For this review, take the finished solid that the model builds, in its own axes (mm). A direction names the side the tool comes from. Round coordinates to 2 decimals unless told otherwise and drop trailing zeros. Write each loop counter-clockwise with the first axis right and the second up, starting at its lowest first coordinate (ties: lowest second). Pieces come first, ordered by that corner, then holes. Notation, with made-up numbers: (16.5, -10) -> (57.5, -10) arc R28 ccw to (57.5, 20) -> close; hole circle Ø3 at (23.25, 20). An arc over 180 degrees is marked (long way). Answer in a Markdown table with one row per item.
from build123d import *

# Parameters (mm, degrees)
SKETCH1_R           = 15.5
BOSS_EXTRUDE1_DEPTH = 2.5
BOSS_EXTRUDE2_DEPTH = 1.9
CIRPATTERN1_COUNT   = 5
BOSS_EXTRUDE3_START = 2.5
SKETCH3_R           = 4.85
BOSS_EXTRUDE3_DEPTH = 2.5
CUT_EXTRUDE2_DEPTH  = 7.9


with BuildPart() as part:
    # Sketch1 → Boss-Extrude1 (new body)
    with BuildSketch(Plane.XY):
        Circle(SKETCH1_R)
    extrude(amount=BOSS_EXTRUDE1_DEPTH)

    # Sketch2 → Boss-Extrude2 (add)
    with BuildSketch(Plane(origin=(0, 0, 0), x_dir=(-1, 0, 0), z_dir=(0, 0, -1))):
        with BuildLine():
            Line((-7.817353518, 8.129035943), (-3.552701535, 4.927044661))
            ThreePointArc((-3.552701535, 4.927044661), (-3.081541521, 4.749426556), (-2.588715364, 4.852685109))
            ThreePointArc((-2.588715364, 4.852685109), (-1.571286021, 5.27077416), (-0.491007267, 5.478039053))
            ThreePointArc((-0.491007267, 5.478039053), (-0.022087339, 5.66148946), (0.274905404, 6.068103848))
            Line((0.274905404, 6.068103848), (2.090121325, 11.082582471))
            ThreePointArc((2.090121325, 11.082582471), (2.007658151, 11.864965509), (1.341576089, 12.283603874))
            ThreePointArc((1.341576089, 12.283603874), (-3.530150602, 11.841654752), (-7.848632729, 9.543883635))
            ThreePointArc((-7.848632729, 9.543883635), (-8.176755455, 8.82885995), (-7.817353518, 8.129035943))
        make_face()
    boss_extrude2 = extrude(amount=BOSS_EXTRUDE2_DEPTH)

    # CirPattern1: Boss-Extrude2 ×5 about axis
    cirpattern1_axis = Axis((0, 0, 0), (0, 0, 1))
    for i in range(1, CIRPATTERN1_COUNT):
        add(boss_extrude2.rotate(cirpattern1_axis, i * 360 / CIRPATTERN1_COUNT))

    # Sketch3 → Boss-Extrude3 (add)
    with BuildSketch(Plane.XY.offset(BOSS_EXTRUDE3_START)):
        Circle(SKETCH3_R)
    extrude(amount=BOSS_EXTRUDE3_DEPTH)

    # Sketch5 → Cut-Extrude2 (cut, through all)
    with BuildSketch(Plane.XY.offset(5)):
        with BuildLine():
            Line((-2.05669638, 1.9), (2.05669638, 1.9))
            ThreePointArc((2.05669638, 1.9), (2.8, 0), (2.05669638, -1.9))
            Line((2.05669638, -1.9), (-2.05669638, -1.9))
            ThreePointArc((-2.05669638, -1.9), (-2.8, 0), (-2.05669638, 1.9))
        make_face()
    extrude(amount=-CUT_EXTRUDE2_DEPTH, mode=Mode.SUBTRACT)


solid = part.part
1) Consider section A-A on y = 0. State the section outline as (x, z) points.
Solved:
| item | result |
|---|---|
| outline | (-15.5, 0) -> (-2.8, 0) -> (-2.8, 5) -> (-4.85, 5) -> (-4.85, 2.5) -> (-15.5, 2.5) -> close; (2.8, 0) -> (5.5, 0) -> (5.5, -1.9) -> (12.36, -1.9) -> (12.36, 0) -> (15.5, 0) -> (15.5, 2.5) -> (4.85, 2.5) -> (4.85, 5) -> (2.8, 5) -> close |
2) Mouldability with a two-part tool opening along Y and no side actions: class faces 1 (the cylindrical face through (4.17, -11.63, -0.94)), 2 (the cylindrical face through (-10.21, 6.96, -0.94)), 3 (the cylindrical face through (-2.018, 15.368, 1.232)), 4 (the flat face through (-0.773, -8.659, -0.937)) as pulls with the +Y half, pulls with the -Y half, needs draft (parallel to the pull), parting line crosses it, or undercut.
Solved:
| item | result |
|---|---|
| face 1 | pulls with the -Y half |
| face 2 | pulls with the +Y half |
| face 3 | parting line crosses it |
| face 4 | undercut |
3) For line 1 (Y direction, x = 6.5, z = -1.5); line 2 (Y direction, x = 0, z = 1.25); line 3 (Y direction, x = -1, z = 4.25), list the stretches that pass through material, from the lowest coordinate up. Write a range as [from, to].
Solved:
| item | result |
|---|---|
| line 1 | [-10.51, -6.58], [-2.36, 2.77], [7.14, 10.51] |
| line 2 | [-15.5, -1.9], [1.9, 15.5] |
| line 3 | [-4.75, -1.9], [1.9, 4.75] |
4) For faces 5 (the flat face through (-4.073, -7.597, -0.937)), 6 (the cylindrical face through (-11.811, -2.346, -0.937)), 7 (the cylindrical face through (2.8, 0, 2.5)), 8 (the cylindrical face through (8.177, 8.84, -0.937)), 9 (the cylindrical face through (3.09, 4.75, -0.94)), list the 3-axis set-ups (+Z, -Z, +X, -X, +Y, -Y) from which the entire face can be reached by the end or side of a thin tool; tool diameter is ignored.
Solved:
| item | result |
|---|---|
| face 5 | -Z, -Y |
| face 6 | -Z, -X |
| face 7 | +Z, -Z |
| face 8 | -Z, +X |
| face 9 | -Z |
5) Clearance check with flat-ended pins moving along their axes: pin 1 Ø1.5 at (y, z) = (7.5, -0.5) entering from -X; pin 2 Ø2 at (x, y) = (-1.5, 4) entering from -Z; pin 3 Ø3 at (x, z) = (-6.5, 2.5) entering from -Y. State where each tip first meets the part, or that it passes through.
Solved:
| item | result |
|---|---|
| pin 1 | x = -13.86 |
| pin 2 | z = 0 |
| pin 3 | y = -14.67 |
6) Consider section B-B on z = 1.25. State the section outline as (x, y) points.
Solved:
| item | result |
|---|---|
| outline | circle Ø31 at (0, 0); hole (-2.06, -1.9) -> (2.06, -1.9) arc R2.8 ccw to (2.06, 1.9) -> (-2.06, 1.9) arc R2.8 ccw to start |
